Autodesk Inventor part; units mm, degrees
ref_plane "Neck Start Plane" through (0, 0, -1.8245) normal (0, 0, 1) x (1, 0, 0)
ref_plane "YZ Plane" through (0, 0, 0) normal (1, 0, 0) x (0, 1, 0)
ref_plane "XZ Plane" through (0, 0, 0) normal (0, 1, 0) x (-1, 0, 0)
ref_plane "Neck Start Plane" through (0, 0, -1.8245) normal (0, 0, 1) x (1, 0, 0)
sketch "Arm Profile" plane through (0, 0, 0) normal (1, 0, 0) x (0, 1, 0)
  line L0 (-2, -0.55) -> (-2, -7.55)
  line L1 (-2, -7.55) -> (-34.3125, -10.9462)
  line L2 (-34.3125, 18.625) -> (-26.7563, 18.625)
  line L3 (-26.692, 18.3928) -> (-31.3125, 15.625)
  arc A0 (-26.692, 18.3928) -> (-26.7563, 18.625) centre (-26.7563, 18.5) ccw
  line L4 (0, 0) -> (-30.5125, 0) construction
  line L5 (-30.5125, 0) -> (-31.3125, 0) construction
  line L6 (-2, -2.9554) -> (-10.1292, -3.3815)
  line L7 (-2, -2.5) -> (-9, -2.8669)
  line L8 (-9, -2.8669) -> (-7.3168, -1.2972)
  line L9 (-7.3168, -1.2972) -> (-2, -0.55)
  line L10 (-10.1292, -3.3815) -> (-31.3125, -5.6079)
  arc A1 (-10.1292, -3.3815) -> (-9, -2.8669) centre (-10.3336, -1.4368) ccw
  line L11 (-2, -2.5) -> (3.8762, -2.192)
  line L12 (3.8762, -2.192) -> (3.9, -2.6462)
  line L13 (3.9, -2.6462) -> (-2, -2.9554)
  line L14 (-31.3125, -5.6079) -> (-31.3125, 15.625)
  line L15 (-34.3125, -10.9462) -> (-34.3125, 18.625)
  line L16 (-31.3125, -5.6079) -> (-31.3125, -10.6309)
  line L17 (-24.5249, -9.9175) -> (-25.047, -4.9494)
  line L18 (-10.1292, -3.3815) -> (-9.607, -8.3495)
  point P0 (-7.4117, -1.3306)
  dimension "d0" = 0.125
  dimension "d1" = 26.7563
  dimension "d2" = 18.5
  dimension "d7" = 3
  dimension "d85" = 2
  dimension "neckDepth" = 7
  dimension "d119" = 30.5125
  dimension "d121" = 0.55
  dimension "d129" = 0.4548
  dimension "d132" = 8
  dimension "d136" = 145
  dimension "d137" = 7
  dimension "d138" = 5.9
  dimension "pincherArmThick" = 3
  dimension "d141" = 0.8
  dimension "d147" = 15
  dimension "d148" = 6
  dimension "d151" = 177
  dimension "d153" = 2.5
extrude "Main Arm" add sketch "Arm Profile" along normal mid plane 9.6 contours L0 L7 L8 L9 | L0 L6 A1 L7 | L0 L1 L18 L6 | L18 L1 L17 L10 | L17 L1 L16 L10
extrude "Pincher" add sketch "Arm Profile" along normal mid plane 11 contours L16 L1 L15 L2 A0 L3 L14
sketch "Neck Sketch" plane through (0, 0, -1.8245) normal (0, 0, 1) x (1, 0, 0)
  line L0 (-1.65, -2) -> (-1.65, 1.1)
  line L1 (-2.85, 3.9) -> (2.85, 3.9)
  line L2 (1.65, 1.1) -> (1.65, -2)
  line L3 (0, -2) -> (0, 3.9) construction
  line L4 (-1.65, 1.1) -> (-2.85, 1.1)
  line L5 (-2.85, 1.1) -> (-2.85, 3.9)
  line L6 (2.85, 3.9) -> (2.85, 1.1)
  line L7 (2.85, 1.1) -> (1.65, 1.1)
  line L8 (1.65, -2) -> (-1.65, -2)
  point P0 (0, 0)
  dimension "neckWidth" = 3.3
  dimension "headWidth" = 5.7
  dimension "headHeight" = 2.8
  dimension "d91" = 2
  dimension "d103" = 1.1
  dimension "neckHeight" = 5.9
extrude "Neck" add sketch "Neck Sketch" against normal blind 5.7255
extrude "Spring Steel Slot" cut sketch "Arm Profile" along normal mid plane 4.9625 contours L11 L12 L13 L0 | L0 L6 A1 L7
extrude "Viewport" cut sketch "Arm Profile" along normal mid plane 4.7625 contours L18 L1 L17 L10
fillet "Fillet1" radius 1.5 5 edges at (-5.15, -31.3125, -10.6309) (5.15, -31.3125, -10.6309) (0, -34.3125, -10.9462) (0, -31.3125, 15.625) (0, -34.3125, 18.625)
fillet "Fillet2" radius 2.3813 4 edges at (-2.3813, -24.7859, -7.4334) (2.3813, -24.7859, -7.4334) (2.3813, -9.8681, -5.8655) (-2.3813, -9.8681, -5.8655)
equation "\"spacing\" = 1"
properties part number "Lever1"
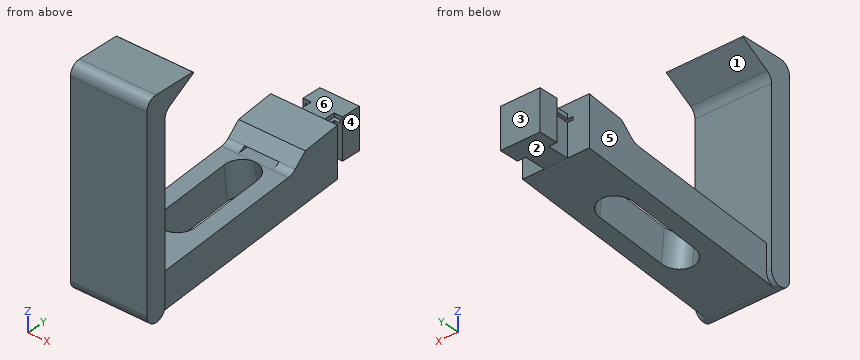
Geometry: final body of the model. Coordinates: model frame, mm. Face numbers are marked on the shaded views. A direction names the side the tool comes from. Round coordinates to 2 decimals unless told otherwise and drop trailing zeros. Order: outer loops, then holes, each group sorted by start corner. A loop starts at its lowest first (then second) coordinate and runs counter-clockwise, first axis right, second up. Notation, with made-up numbers: (4.5, -8.75) -> (33.5, -8.75) arc R36 ccw to (33.5, 30.25) -> close; hole circle Ø9 at (29, -15.75). An arc over 180 degrees is marked (long way). Use CSV: the item, a comma, the result in double quotes. Start each with the question number.
1) Section C-C (z = 7.75). Return the cut outline in (x, y).
2) Set-up query: the marked faces 4, 5 and 6. Return all of +Z, -Z, +X, -X, +Y, -Y with unobstructed straight access to the full face (end or side cutting, diameter ignored); none if empty.
3) Material intervals for line 1 along X through (y, z) = (-20.5, -5); line 2 along Y through (x, z) = (-0.5, 9.5); line 3 along Y through (x, z) = (1.5, -7), sorted ascending. Write a range as from..to.
4) Draft query along Z for the marked faces 1, 2 and 3. Return one class per face: +Z half, -Z half, draft (parallel to the pull), parting line (faces both ways), or undercut.
5) Section D-D (y = -17). Return the cut outline in (x, z).
6) Section B-B (y = -3). Return the cut outline in (x, z).
7) Section A-A (y = -29). Return the cut outline in (x, z) (3 decimals), and give its area (3 significant figures).
8) First-contact query: pin 1 Ø3.5 at (y, z) = (-1, -5) entering from -X; pin 2 Ø0.7 at (y, z) = (0, -2) entering from -X; pin 3 Ø1 at (y, z) = (-6.5, -3) entering from +X. Flat tips, straight axial feed; report the tip coordinate or a pass-through.
Returned:
1,outline,"(-5.5, -34.31) -> (5.5, -34.31) -> (5.5, -31.31) -> (-5.5, -31.31) -> close"
2,face 4,"+Z, -Z, +X, +Y"
2,face 5,"-Z, -X, +Y"
2,face 6,"+Z, +X, -X, +Y"
3,line 1,"x = -4.8..-2.38, 2.38..4.8"
3,line 2,"y = -34.31..-31.31"
3,line 3,"y = -34.31..-24.3, -10.28..3.9"
4,face 1,"undercut"
4,face 2,"-Z half"
4,face 3,"draft"
5,outline,"(-4.8, -9.13) -> (-2.38, -9.13) -> (-2.38, -4.1) -> (-4.8, -4.1) -> close; (2.38, -9.13) -> (4.8, -9.13) -> (4.8, -4.1) -> (2.38, -4.1) -> close"
6,outline,"(-4.8, -7.66) -> (4.8, -7.66) -> (4.8, -0.69) -> (-4.8, -0.69) -> close; hole (-2.48, -3.01) -> (2.48, -3.01) -> (2.48, -2.55) -> (-2.48, -2.55) -> close"
7,outline,"(-5.5, 17.01) -> (5.5, 17.01) -> (5.5, 18.625) -> (-5.5, 18.625) -> close; (-4.8, -10.388) -> (4.8, -10.388) -> (4.8, -5.365) -> (-4.8, -5.365) -> close"
7,area,"66.0 mm²"
8,pin 1,"stops at x = -4.8"
8,pin 2,"stops at x = -1.65"
8,pin 3,"stops at x = 4.8"
